Verification items for the finished model (mm, model axes). Round coordinates to 2 decimals unless told otherwise and drop trailing zeros. Loops run counter-clockwise (first coordinate to the right, second up) from the corner with the lowest first, then second, coordinate; pieces in that order, holes last. Notation, with made-up numbers: M 37,64 L 42,64 A23 ccw 42,99 Z; hole C 33.25,46.5 d7. An arc over 180 degrees is marked long. Answer as CSV lines item,"result".
Autodesk Inventor part; units mm, degrees
ref_plane "YZ Plane" through (0, 0, 0) normal (1, 0, 0) x (0, 1, 0)
ref_plane "XZ Plane" through (0, 0, 0) normal (0, 1, 0) x (-1, 0, 0)
ref_plane "XY Plane" through (0, 0, 0) normal (0, 0, 1) x (1, 0, 0)
sketch "Sketch1" plane through (0, 0, 0) normal (0, 0, 1) x (1, 0, 0)
  line L0 (3.175, 0) -> (22.225, 0)
  line L1 (25.4, 3.175) -> (25.4, 22.225)
  line L2 (22.225, 25.4) -> (3.175, 25.4)
  line L3 (0, 22.225) -> (0, 3.175)
  arc A0 (3.175, 25.4) -> (0, 22.225) centre (3.175, 22.225) ccw
  arc A1 (0, 3.175) -> (3.175, 0) centre (3.175, 3.175) ccw
  arc A2 (22.225, 0) -> (25.4, 3.175) centre (22.225, 3.175) ccw
  arc A3 (25.4, 22.225) -> (22.225, 25.4) centre (22.225, 22.225) ccw
  line L4 (3.175, 23.4) -> (22.225, 23.4)
  arc A4 (23.4, 22.225) -> (22.225, 23.4) centre (22.225, 22.225) ccw
  line L5 (23.4, 22.225) -> (23.4, 3.175)
  arc A5 (22.225, 2) -> (23.4, 3.175) centre (22.225, 3.175) ccw
  line L6 (22.225, 2) -> (3.175, 2)
  arc A6 (2, 3.175) -> (3.175, 2) centre (3.175, 3.175) ccw
  line L7 (2, 3.175) -> (2, 22.225)
  arc A7 (3.175, 23.4) -> (2, 22.225) centre (3.175, 22.225) ccw
  point P0 (0, 0)
  point P1 (25.4, 0)
  point P2 (0, 25.4)
  dimension "d0" = 25.4
  dimension "d1" = 25.4
  dimension "d2" = 3.175
  dimension "d3" = 2
extrude "Extrusion1" add sketch "Sketch1" along normal blind 1000
sketch "Sketch11" plane through (3.175, 25.4, 1000) normal (0, 1, 0) x (1, 0, 0)
  circle A0 centre (9.525, 500) radius 4.7917
  point P0 (-3.175, 1000)
hole "centerHole" at (12.7, 25.4, 500) direction (0, -1, 0) diameter 11 end through all
sketch "Sketch12" plane through (3.175, 25.4, 1000) normal (0, 1, 0) x (1, 0, 0)
  line L0 (0, 1000) -> (0, 0)
  circle A0 centre (9.525, 927) radius 1.5875
  circle A1 centre (9.525, 777) radius 1.5875
  circle A2 centre (9.525, 627) radius 1.5875
  circle A3 centre (9.525, 500) radius 5.5
  point P0 (-3.175, 1000)
  dimension "d76" = 3.175
  dimension "d80" = 150
  dimension "d140" = 127
hole "longSideHoles" at (12.7, 25.4, 73) at (12.7, 25.4, 223) at (12.7, 25.4, 373) direction (0, -1, 0) diameter 5.5 end through all
sketch "Sketch13" plane through (3.175, 25.4, 1000) normal (0, 1, 0) x (1, 0, 0)
  line L0 (0, 1000) -> (0, 0)
  circle A0 centre (9.525, 68.2) radius 1.5875
  circle A1 centre (9.525, 220.6) radius 1.5875
  circle A2 centre (9.525, 373) radius 1.5875
  circle A3 centre (9.525, 500) radius 5.5
  point P0 (-3.175, 1000)
  dimension "d96" = 152.4
  dimension "d137" = 127
  dimension "d138" = 152.4
hole "shortSideHoles" at (12.7, 25.4, 627) at (12.7, 25.4, 779.4) at (12.7, 25.4, 931.8) direction (0, -1, 0) diameter 5.5 end through all
sketch "Sketch14" plane through (25.4, 22.225, 1000) normal (1, 0, 0) x (0, 0, -1)
  line L0 (1000, -19.05) -> (1000, 0)
  line L1 (0, -19.05) -> (0, 0)
  circle A0 centre (30, -9.525) radius 4.7625
  circle A1 centre (980, -9.525) radius 4.7625
  point P0 (1000, -22.225)
  dimension "d108" = 9.525
  dimension "d109" = 30
  dimension "d110" = 9.525
  dimension "d111" = 20
hole "shackleHole" at (25.4, 12.7, 970) at (25.4, 12.7, 20) direction (-1, 0, 0) diameter 8 end through all
sketch "Sketch15" plane through (3.175, 25.4, 1000) normal (0, 1, 0) x (1, 0, 0)
  circle A0 centre (9.525, 500) radius 5.5
  circle A1 centre (9.525, 560) radius 3.175
  point P0 (-3.175, 1000)
  dimension "d119" = 6.35
  dimension "d120" = 60
hole "collarHole" at (12.7, 25.4, 440) direction (0, -1, 0) diameter 6.6 end through all
sketch "Sketch16" plane through (0, 0, 1000) normal (0, 0, 1) x (1, 0, 0)
  arc A0 (23.4, 22.225) -> (22.225, 23.4) centre (22.225, 22.225) ccw
  line L0 (23.4, 22.225) -> (23.4, 3.175)
  arc A1 (22.225, 2) -> (23.4, 3.175) centre (22.225, 3.175) ccw
  line L1 (22.225, 2) -> (3.175, 2)
  arc A2 (2, 3.175) -> (3.175, 2) centre (3.175, 3.175) ccw
  line L2 (2, 3.175) -> (2, 22.225)
  arc A3 (3.175, 23.4) -> (2, 22.225) centre (3.175, 22.225) ccw
  line L3 (3.175, 23.4) -> (22.225, 23.4)
  line L4 (0, 22.225) -> (0, 3.175)
  arc A4 (0, 3.175) -> (3.175, 0) centre (3.175, 3.175) ccw
  line L5 (3.175, 0) -> (22.225, 0)
  arc A5 (22.225, 0) -> (25.4, 3.175) centre (22.225, 3.175) ccw
  line L6 (25.4, 3.175) -> (25.4, 22.225)
  arc A6 (25.4, 22.225) -> (22.225, 25.4) centre (22.225, 22.225) ccw
  line L7 (22.225, 25.4) -> (3.175, 25.4)
  arc A7 (3.175, 25.4) -> (0, 22.225) centre (3.175, 22.225) ccw
  point P0 (0, 0)
extrude "removeSide" cut sketch "Sketch16" against normal blind 195
equation "\"tube\" = 25.4"
properties part number "2f2al" material "Steel"
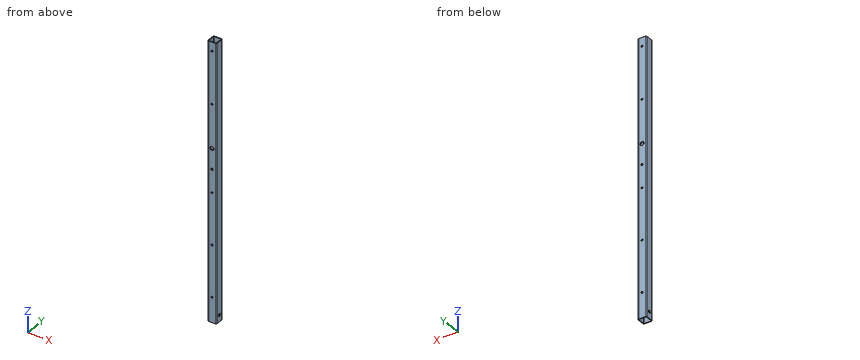
1) Material ranges on probe 1 along Y at (x, z) = (6.5, 167); probe 2 along Y at (x, z) = (2.75, 138), recorded low to high.
Here are the results:
probe 1,"y = 0 to 2, 23.4 to 25.4"
probe 2,"y = 0.03 to 2.08, 23.32 to 25.37"
2) Go/stop test with a flat-tipped pin: pin 1 (5.5 mm diameter, centred on x = 12.7, z = 440, fed in from +Y). Record where the tip stops, or that it passes through.
Here are the results:
pin 1,"passes through"
3) Section check A-A (z = 408.5). Record the cut outline in (x, y) (3 decimals), plus the area to 3 significant figures.
Here are the results:
outline,"M 0,3.175 A3.175 ccw 3.175,0 L 22.225,0 A3.175 ccw 25.4,3.175 L 25.4,22.225 A3.175 ccw 22.225,25.4 L 3.175,25.4 A3.175 ccw 0,22.225 Z; hole M 2,3.175 A1.175 ccw 3.175,2 L 22.225,2 A1.175 ccw 23.4,3.175 L 23.4,22.225 A1.175 ccw 22.225,23.4 L 3.175,23.4 A1.175 ccw 2,22.225 Z"
area,"180 mm^2"
